Geometry: final body of the model. Coordinates: model frame, mm. A direction names the side the tool comes from. Round coordinates to 2 decimals unless told otherwise and drop trailing zeros. Order: outer loops, then holes, each group sorted by start corner. A loop starts at its lowest first (then second) coordinate and runs counter-clockwise, first axis right, second up. Notation, with made-up numbers: (52.5, -36.5) - (87.5, -36.5) arc R11 cw to (87.5, -25.5) - close; hole circle Ø4 at (-8.5, 64). An arc over 180 degrees is marked (long way). Put each result on its own line as item: value. Start each with the question number.
(1) Access query for faces 4 (the face through (-23, 9, -68)), 5 (the face through (-1, 0, -1)). Directions: +Z, -Z, +X, -X, +Y, -Y. A direction counts if a zero-diameter tool reaches every point of the face in a straight line with its end or side. Return the directions, or none.
(2) Material intervals for L1, parallel to Z at x = -23, y = 9.35; L2, parallel to Z at x = -23, y = 9.65; L3, parallel to X at y = 9.65, z = -68, sorted ascending. Write a range as [from, to].
(3) Section A-A (z = -68). Output: boundary loops of the cut face in (x, y).
(4) Pull-direction query (Z, two-part tool) for faces 1 (the face through (39, 5, -83)), 2 (the face through (-28.952, 9.507, -63.436)), 3 (the face through (38, 5, 84)); classes: released by +Z, released by -Z, zero draft, split by the parting line, or undercut.
from build123d import *

# Parameters (mm, degrees)
SKETCH1_W           = 80
SKETCH1_H           = 170
BOSS_EXTRUDE1_DEPTH = 10
FILLET4_R           = 5
FILLET5_R           = 2
SKETCH3_R           = 7.5
CUT_EXTRUDE1_DEPTH  = 1


with BuildPart() as part:
    # Sketch1 → Boss-Extrude1 (new body)
    with BuildSketch(Plane(origin=(0, 0, 0), x_dir=(1, 0, 0), z_dir=(0, 1, 0))):
        Rectangle(SKETCH1_W, SKETCH1_H)
    extrude(amount=BOSS_EXTRUDE1_DEPTH)

    # Fillet4
    fillet4_edges = [part.edges().sort_by_distance(p)[0] for p in [
        (40, 5, 85),
        (-40, 5, 85),
        (-40, 5, -85),
        (40, 5, -85),
    ]]
    fillet(fillet4_edges, radius=FILLET4_R)

    # Fillet5
    fillet5_edges = [part.edges().sort_by_distance(p)[0] for p in [
        (0, 0, -85),
        (0, 10, -85),
        (40, 0, 0),
        (0, 0, 85),
        (-40, 0, 0),
        (38.535533906, 0, 83.535533906),
        (-38.535533906, 0, 83.535533906),
        (-38.535533906, 0, -83.535533906),
        (38.535533906, 0, -83.535533906),
        (40, 10, 0),
        (-40, 10, 0),
        (0, 10, 85),
        (38.535533906, 10, 83.535533906),
        (-38.535533906, 10, 83.535533906),
        (-38.535533906, 10, -83.535533906),
        (38.535533906, 10, -83.535533906),
    ]]
    fillet(fillet5_edges, radius=FILLET5_R)

    # Sketch3 → Cut-Extrude1 (cut)
    with BuildSketch(Plane(origin=(0, 10, 0), x_dir=(1, 0, 0), z_dir=(0, 1, 0))):
        with Locations((-23, 68)):
            Circle(SKETCH3_R)
    extrude(amount=-CUT_EXTRUDE1_DEPTH, mode=Mode.SUBTRACT)


solid = part.part
Checks:
1. face 4: +Y
1. face 5: +Z, -Z, +X, -X, -Y
2. L1: z = [-84.48, -75.5], [-60.5, 84.48]
2. L2: z = [-84.13, -75.5], [-60.5, 84.13]
2. L3: x = [-39.13, -30.5], [-15.5, 39.13]
3. outline: (-40, 2) arc R2 ccw to (-38, 0) - (38, 0) arc R2 ccw to (40, 2) - (40, 8) arc R2 ccw to (38, 10) - (-15.5, 10) - (-15.5, 9) - (-30.5, 9) - (-30.5, 10) - (-38, 10) arc R2 ccw to (-40, 8) - close
4. face 1: released by -Z
4. face 2: undercut
4. face 3: released by +Z
